from build123d import *

# Parameters (mm, degrees)
BOSS_EXTRUDE1_DEPTH  = 6
M8_CLEARANCE_HOLE1_D = 9
SKETCH5_R            = 5
CUT_EXTRUDE1_DEPTH   = 105.575331699


with BuildPart() as part:
    # Sketch1 → Boss-Extrude1 (new body)
    with BuildSketch(Plane.XY):
        Polygon((0, 100), (30, 100), (30, -50), (-6, -50), (-6, 0), (0, 0), align=None)
    extrude(amount=BOSS_EXTRUDE1_DEPTH)

    # M8 Clearance Hole1 (through all)
    with Locations(Plane.XY.offset(6)):
        with Locations((15, 62.5), (15, 25), (15, -12.5)):
            Hole(M8_CLEARANCE_HOLE1_D / 2)

    # Sketch5 → Cut-Extrude1 (cut, through all)
    with BuildSketch(Plane(origin=(0, 0, 0), x_dir=(-1, 0, 0), z_dir=(0, 0, -1))):
        with Locations((0, 5)):
            Circle(SKETCH5_R)
    extrude(amount=-CUT_EXTRUDE1_DEPTH, mode=Mode.SUBTRACT)


solid = part.part
Geometry: final body of the model. Coordinates: model frame, mm. A direction names the side the tool comes from. Round coordinates to 2 decimals unless told otherwise and drop trailing zeros. Loops run counter-clockwise (first coordinate to the right, second up) from the corner with the lowest first, then second, coordinate; pieces in that order, holes last.
Q1. Section D-D on y = 25. Return loops of the section in (x, z), plus the area to 3 significant figures.
Q2. Pin query (flat end, axial travel): P1, Ø2, axis at y = 53, z = 4, coming from the -X side. Return the tip coordinate at first contact, or that it passes through.
Q3. Section B-B on x = 15. Return loops of the section in (y, z).
Q4. Pull-direction query (X, two-part tool) for faces 1 (the flat face through (30, 26, 3)), 2 (the cylindrical face through (19.496, -12.302, 2.958)), 3 (the flat face through (-6, -25, 3)), 4 (the flat face through (15, 100, 3)); classes: released by +X, released by -X, zero draft, split by the parting line, or undercut.
Q5. Access query for faces 5 (the flat face through (-3, 0, 3)), 6 (the flat face through (8, 26, 0)). Directions: +Z, -Z, +X, -X, +Y, -Y. A direction counts if a zero-diameter tool reaches every point of the face in a straight line with its end or side. Return the directions, or none.
Q6. Section A-A on y = -12.5. Return loops of the section in (x, z), plus the area to 3 significant figures.
Q7. Material intervals for L1, parallel to Y at x = 15, z = 4.75; L2, parallel to Y at x = 19, z = 4.5; L3, parallel to X at y = -13, z = 0.35, sorted ascending.
Q8. Section C-C on z = 3.6. Return loops of the section in (x, y).
Evaluation:
1. outline: (0, 0) - (10.5, 0) - (10.5, 6) - (0, 6) - close; (19.5, 0) - (30, 0) - (30, 6) - (19.5, 6) - close
1. area: 126 mm2
2. P1: stops at x = 0
3. outline: (-50, 0) - (-17, 0) - (-17, 6) - (-50, 6) - close; (-8, 0) - (20.5, 0) - (20.5, 6) - (-8, 6) - close; (29.5, 0) - (58, 0) - (58, 6) - (29.5, 6) - close; (67, 0) - (100, 0) - (100, 6) - (67, 6) - close
4. face 1: released by +X
4. face 2: undercut
4. face 3: released by -X
4. face 4: zero draft
5. face 5: +Z, -Z, -X, +Y
5. face 6: -Z, +X, -X, +Y, -Y
6. outline: (-6, 0) - (10.5, 0) - (10.5, 6) - (-6, 6) - close; (19.5, 0) - (30, 0) - (30, 6) - (19.5, 6) - close
6. area: 162 mm2
7. L1: y = -50 to -17, -8 to 20.5, 29.5 to 58, 67 to 100
7. L2: y = -50 to -14.56, -10.44 to 22.94, 27.06 to 60.44, 64.56 to 100
7. L3: x = -6 to 10.53, 19.47 to 30
8. outline: (-6, -50) - (30, -50) - (30, 100) - (0, 100) - (0, 10) arc R5 cw to (0, 0) - (-6, 0) - close; hole circle Ø9 at (15, -12.5); hole circle Ø9 at (15, 25); hole circle Ø9 at (15, 62.5)
